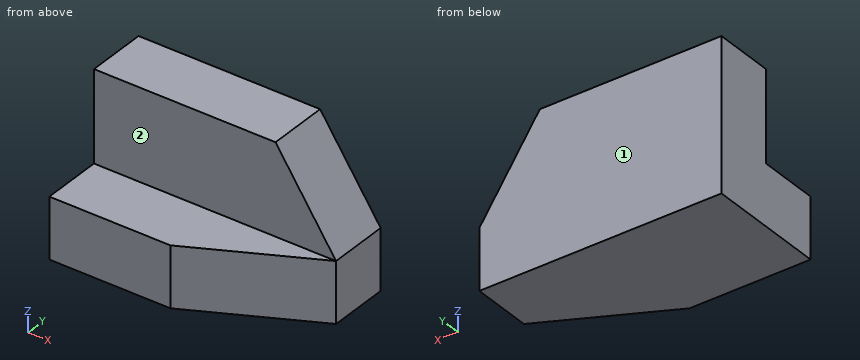
```python
from build123d import *

# Parameters (mm, degrees)
F0_W     = 50.8
F0_H     = 31.75
F1_DEPTH = 25.4
F2_W     = 50.8
F2_H     = 19.05
F3_DEPTH = 12.7
F5_DEPTH = 25.4
F7_DEPTH = 25.4


with BuildPart() as f1:
    # F0 (on Front) → F1 (new body)
    with BuildSketch(Plane.XZ):
        with Locations((25.4, 15.875)):
            Rectangle(F0_W, F0_H)
    extrude(amount=F1_DEPTH)

    # F2 (on face) → F3 (cut)
    with BuildSketch(Plane.XZ.offset(25.4)):
        with Locations((25.4, 22.225)):
            Rectangle(F2_W, F2_H)
    extrude(amount=-F3_DEPTH, mode=Mode.SUBTRACT)

    # F4 (on face) → F5 (cut)
    with BuildSketch(Plane.XY.offset(12.7)):
        Polygon((50.8, -25.4), (50.8, -12.7), (25.4, -25.4), align=None)
    extrude(amount=-F5_DEPTH, mode=Mode.SUBTRACT)

    # F6 (on face) → F7 (cut)
    with BuildSketch(Plane.XZ.offset(12.7)):
        Polygon((38.1, 31.75), (50.8, 12.7), (50.8, 31.75), align=None)
    extrude(amount=-F7_DEPTH, mode=Mode.SUBTRACT)


solid = f1.part
```
The listing builds one solid part. Answer for the finished solid, in the listing's coordinates (mm). Face numbers are marked on the shaded views. A direction names the side the tool comes from. Give positions to 0.01 mm unless a question says otherwise; leave off trailing zeros. Write each loop counter-clockwise with the first axis right and the second up, starting at its lowest first coordinate (ties: lowest second). Pieces come first, ordered by that corner, then holes. Notation, with made-up numbers: (32.25, 86) -> (48.25, 86) arc R21 cw to (48.25, 96) -> close; hole circle Ø4 at (-23.5, 28). An arc over 180 degrees is marked (long way). Use one line per item in the form item = value.
1) Section C-C on z = 9 is taken. Write down the section's boundary in (x, y).
Result:
outline = (0, -25.4) -> (25.4, -25.4) -> (50.8, -12.7) -> (50.8, 0) -> (0, 0) -> close
2) Each of these flat-tipped pins is pushed along its axis until it touches: P1, Ø10, axis at y = -17.5, z = 8, coming from the +X side; P2, Ø4, axis at x = 32, y = -22, coming from the +Z side; P3, Ø3, axis at x = 35.5, z = 12, coming from the -Y side; P4, Ø5, axis at x = 20, z = 27, coming from the -Y side. Where does it stop, or does it pass through?
Result:
P1 = 50.8
P2 = 12.7
P3 = -21.1
P4 = -12.7
3) Section B-B on y = -10.25 is taken. Write down the section's boundary in (x, z), plus the area to 3 significant figures.
Result:
outline = (0, 0) -> (50.8, 0) -> (50.8, 12.7) -> (38.1, 31.75) -> (0, 31.75) -> close
area = 1,490 mm²
4) Section A-A on x = 18 is taken. Write down the section's boundary in (y, z), plus the area to 3 significant figures.
Result:
outline = (-25.4, 0) -> (0, 0) -> (0, 31.75) -> (-12.7, 31.75) -> (-12.7, 12.7) -> (-25.4, 12.7) -> close
area = 565 mm²
5) Section D-D on x = 31 is taken. Write down the section's boundary in (y, z), plus the area to 3 significant figures.
Result:
outline = (-22.6, 0) -> (0, 0) -> (0, 31.75) -> (-12.7, 31.75) -> (-12.7, 12.7) -> (-22.6, 12.7) -> close
area = 529 mm²
6) A tool of negligible diameter and unlimited length cuts with its end or side. For the marked faces 1 and 2, from which of +Z, -Z, +X, -X, +Y, -Y can it reach the whole face along a straight path? Write none if from no direction.
Result:
face_1 = +Z, -Z, +X, -X, +Y
face_2 = +Z, +X, -X, -Y
7) Straight lines are drawn through the part: probe 1 along Y at (x, z) = (12, 15); probe 2 along Z at (x, y) = (37, -19.25); probe 3 along Z at (x, y) = (40, -5.5). For each, find the intervals that lie inside material, in ascending order.
Result:
probe_1 = -12.7 to 0
probe_2 = 0 to 12.7
probe_3 = 0 to 28.9
